from build123d import *

# Parameters (mm, degrees)
BOSS_EXTRUDE1_DEPTH = 45
SKETCH2_W           = 78
SKETCH2_H           = 38
CUT_EXTRUDE1_DEPTH  = 17
CUT_EXTRUDE2_REACH  = 130.949
SKETCH3_W           = 72
SKETCH3_H           = 32
FILLET1_R           = 10
FILLET2_R           = 7
CUT_EXTRUDE3_REACH  = 97.222
SKETCH4_W           = 18
SKETCH4_H           = 15
CUT_EXTRUDE4_REACH  = 131.379
SKETCH5_R           = 1.6


with BuildPart() as part:
    # Sketch1 → Boss-Extrude1 (new body)
    with BuildSketch(Plane.XY):
        Polygon((34.641016151, 20), (3, 1.732050808), (4, 0), (119.641016151, 0), (119.641016151, 20), align=None)
    extrude(amount=BOSS_EXTRUDE1_DEPTH)

    # Sketch2 → Cut-Extrude1 (cut)
    with BuildSketch(Plane(origin=(0, 20, 0), x_dir=(1, 0, 0), z_dir=(0, 1, 0))):
        with Locations((77.141016151, -22.5)):
            Rectangle(SKETCH2_W, SKETCH2_H)
    extrude(amount=-CUT_EXTRUDE1_DEPTH, mode=Mode.SUBTRACT)

    # Sketch3 → Cut-Extrude2 (cut, up to next)
    with BuildSketch(Plane(origin=(0, 3, 0), x_dir=(1, 0, 0), z_dir=(0, 1, 0)), mode=Mode.PRIVATE) as cut_extrude2_sk1:
        with Locations((77.141016151, -22.5)):
            Rectangle(SKETCH3_W, SKETCH3_H)
    cut_extrude2_tool1 = extrude(cut_extrude2_sk1.sketch, amount=-CUT_EXTRUDE2_REACH, mode=Mode.PRIVATE) & part.part
    add(cut_extrude2_tool1.solids().sort_by_distance((77.141016, 3, 22.5))[0], mode=Mode.SUBTRACT)

    # Fillet1
    fillet1_edges = [part.edges().sort_by_distance(p)[0] for p in [
        (119.641016151, 10, 45),
        (119.641016151, 10, 0),
    ]]
    fillet(fillet1_edges, radius=FILLET1_R)

    # Fillet2
    fillet2_edges = [part.edges().sort_by_distance(p)[0] for p in [
        (41.141016151, 1.5, 38.5),
        (41.141016151, 1.5, 6.5),
        (113.141016151, 1.5, 6.5),
        (113.141016151, 1.5, 38.5),
    ]]
    fillet(fillet2_edges, radius=FILLET2_R)

    # Cut-Extrude3: up to this plane
    cut_extrude3_end = Plane(origin=(0, 0, 45), z_dir=(-0.5000000000000014, 0.8660254037844379, 0))
    # Sketch4 → Cut-Extrude3 (cut, up to the surface)
    with BuildSketch(Plane(origin=(38.141016151, 0, 0), x_dir=(0, 0, -1), z_dir=(1, 0, 0)), mode=Mode.PRIVATE) as cut_extrude3_sk1:
        with Locations((-22.5, 10.5)):
            Rectangle(SKETCH4_W, SKETCH4_H)
    cut_extrude3_tool1 = split(extrude(cut_extrude3_sk1.sketch, amount=-CUT_EXTRUDE3_REACH, mode=Mode.PRIVATE), bisect_by=cut_extrude3_end, keep=Keep.BOTH, mode=Mode.PRIVATE)
    add(cut_extrude3_tool1.solids().sort_by_distance((38.141016, 10.5, 22.5))[0], mode=Mode.SUBTRACT)

    # Cut-Extrude4: up to this plane
    cut_extrude4_end = Plane(origin=(0, 2, 45), z_dir=(0, 1, 0))
    # Sketch5 → Cut-Extrude4 (cut, up to the surface)
    with BuildSketch(Plane(origin=(0, 0, 0), x_dir=(0.8660254037844378, 0.5000000000000017, 0), z_dir=(-0.5000000000000016, 0.8660254037844377, 0)), mode=Mode.PRIVATE) as cut_extrude4_sk1:
        with Locations(Location((13.464101615, -5, 0), (0, 0, 180))):
            Circle(SKETCH5_R)
    cut_extrude4_tool1 = split(extrude(cut_extrude4_sk1.sketch, amount=-CUT_EXTRUDE4_REACH, mode=Mode.PRIVATE), bisect_by=cut_extrude4_end, keep=Keep.BOTH, mode=Mode.PRIVATE)
    add(cut_extrude4_tool1.solids().sort_by_distance((11.660254, 6.732051, 5))[0], mode=Mode.SUBTRACT)
    # Sketch5 → Cut-Extrude4 (cut, up to the surface)
    with BuildSketch(Plane(origin=(0, 0, 0), x_dir=(0.8660254037844378, 0.5000000000000017, 0), z_dir=(-0.5000000000000016, 0.8660254037844377, 0)), mode=Mode.PRIVATE) as cut_extrude4_sk2:
        with Locations(Location((13.464101615, -40, 0), (0, 0, 180))):
            Circle(SKETCH5_R)
    cut_extrude4_tool2 = split(extrude(cut_extrude4_sk2.sketch, amount=-CUT_EXTRUDE4_REACH, mode=Mode.PRIVATE), bisect_by=cut_extrude4_end, keep=Keep.BOTH, mode=Mode.PRIVATE)
    add(cut_extrude4_tool2.solids().sort_by_distance((11.660254, 6.732051, 40))[0], mode=Mode.SUBTRACT)


solid = part.part
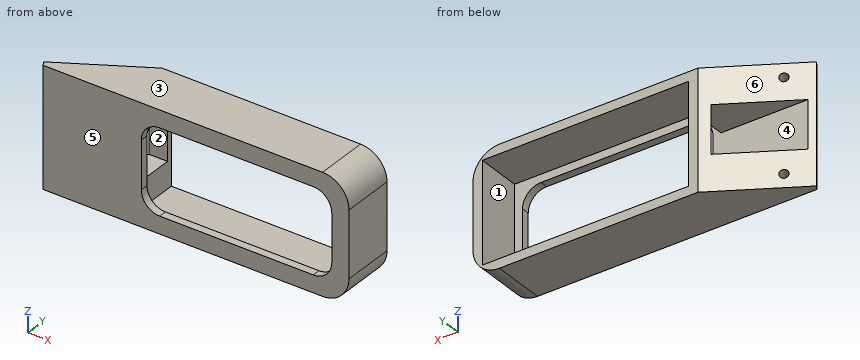
Source: CAD feature listing. Evaluate the final solid. Frame: model axes, mm. Face numbers are marked on the shaded views. A direction names the side the tool comes from. Round coordinates to 2 decimals unless told otherwise and drop trailing zeros. Loops run counter-clockwise (first coordinate to the right, second up) from the corner with the lowest first, then second, coordinate; pieces in that order, holes last.
Q1. Ray query, line 1 (Z direction, x = 47.5, y = 17.25); line 2 (X direction, y = 7.25, z = 11); line 3 (Z direction, x = 35.5, y = 9.5). Return the intervals inside material, ascending.
Q2. Mould query, pull axis X, two halves, no side actions, for the marked faces 4, 5 and 6. Classes: pulls with the +X half, pulls with the -X half, needs draft (parallel to the pull), parting line crosses it, or undercut.
Q3. First-contact query: P1, Ø5, axis at y = 13, z = 8, coming from the -X side; P2, Ø6, axis at x = 17, z = 15, coming from the -Y side; P3, Ø1.6, axis at x = 15, z = 40, coming from the +Y side; P4, Ø3.5, axis at x = 15, z = 5.5, coming from the +Y side. Flat tips, straight axial feed; report the tip coordinate or a pass-through.
Q4. Section D-D, the plane y = 12.25. Return loops of the section in (x, z).
Q5. Section A-A, the plane x = 56.5. Return loops of the section in (y, z), plus the area to 3 significant figures.
Q6. Section B-B, the plane z = 17. Return loops of the section in (x, y).
Q7. Access query for the marked faces 1, 2 and 3. Directions: +Z, -Z, +X, -X, +Y, -Y. A direction counts if a zero-diameter tool reaches every point of the face in a straight line with its end or side. Return the directions, or none.
Q8. Section C-C, the plane z = 33.5. Return loops of the section in (x, y).
Solutions:
1. line 1: z = 0 to 3.5, 41.5 to 45
1. line 2: x = 12.56 to 38.14, 116.14 to 119.64
1. line 3: z = 0 to 13.5, 31.5 to 45
2. face 4: undercut
2. face 5: needs draft
2. face 6: pulls with the -X half
3. P1: stops at x = 18.19
3. P2: stops at y = 0
3. P3: stops at y = 9.12
3. P4: stops at y = 9.67
4. outline: (21.22, 0) - (109.64, 0) arc R10 ccw to (119.64, 10) - (119.64, 35) arc R10 ccw to (109.64, 45) - (21.22, 45) - (21.22, 31.5) - (38.14, 31.5) - (38.14, 41.5) - (116.14, 41.5) - (116.14, 3.5) - (38.14, 3.5) - (38.14, 13.5) - (21.22, 13.5) - close
5. outline: (0, 0) - (20, 0) - (20, 3.5) - (3, 3.5) - (3, 6.5) - (0, 6.5) - close; (0, 38.5) - (3, 38.5) - (3, 41.5) - (20, 41.5) - (20, 45) - (0, 45) - close
5. area: 158 mm2
6. outline: (3, 1.73) - (4, 0) - (41.14, 0) - (41.14, 3) - (5.2, 3) - close; (31.18, 18) - (38.14, 18) - (38.14, 20) - (34.64, 20) - close; (113.14, 0) - (119.64, 0) - (119.64, 20) - (116.14, 20) - (116.14, 3) - (113.14, 3) - close
7. face 1: +Y
7. face 2: -X
7. face 3: +Z, +X, -X, +Y, -Y
8. outline: (3, 1.73) - (4, 0) - (41.43, 0) - (41.43, 3) - (38.14, 3) - (38.14, 20) - (34.64, 20) - close; (112.85, 0) - (119.64, 0) - (119.64, 20) - (116.14, 20) - (116.14, 3) - (112.85, 3) - close
